```python
from build123d import *

# Parameters (mm, degrees)
F0_W     = 228.6
F0_H     = 88.9
F1_DEPTH = 1.27
F2_R     = 12.7
F4_DEPTH = 25.4
F6_DEPTH = 1.271


with BuildPart() as f1:
    # F0 (on Top) → F1 (new body)
    with BuildSketch(Plane.XY):
        with Locations((114.3, 44.45)):
            Rectangle(F0_W, F0_H)
    extrude(amount=F1_DEPTH)

    # F2
    f2_edges = [f1.edges().sort_by_distance(p)[0] for p in [
        (228.6, 0, 0.635),
        (228.6, 88.9, 0.635),
        (0, 88.9, 0.635),
        (0, 0, 0.635),
    ]]
    fillet(f2_edges, radius=F2_R)

    # F3 (on face) → F4 (cut)
    with BuildSketch(Plane.XY.offset(1.27)):
        with BuildLine():
            Line((44.45, 16.2687), (6.35, 16.2687))
            ThreePointArc((6.35, 16.2687), (2.7813, 12.7), (6.35, 9.1313))
            Line((6.35, 9.1313), (44.45, 9.1313))
            ThreePointArc((44.45, 9.1313), (48.0187, 12.7), (44.45, 16.2687))
        make_face()
        with BuildLine():
            ThreePointArc((6.35, 79.7687), (2.7813, 76.2), (6.35, 72.6313))
            Line((6.35, 72.6313), (44.45, 72.6313))
            ThreePointArc((44.45, 72.6313), (48.0187, 76.2), (44.45, 79.7687))
            Line((44.45, 79.7687), (6.35, 79.7687))
        make_face()
        with BuildLine():
            ThreePointArc((222.25, 72.6313), (225.8187, 76.2), (222.25, 79.7687))
            Line((222.25, 79.7687), (184.15, 79.7687))
            ThreePointArc((184.15, 79.7687), (180.5813, 76.2), (184.15, 72.6313))
            Line((184.15, 72.6313), (222.25, 72.6313))
        make_face()
        with BuildLine():
            ThreePointArc((222.25, 9.1313), (225.8187, 12.7), (222.25, 16.2687))
            Line((222.25, 16.2687), (184.15, 16.2687))
            ThreePointArc((184.15, 16.2687), (180.5813, 12.7), (184.15, 9.1313))
            Line((184.15, 9.1313), (222.25, 9.1313))
        make_face()
    extrude(amount=-F4_DEPTH, mode=Mode.SUBTRACT)

    # F5 (on face) → F6 (cut, through all)
    with BuildSketch(Plane.XY.offset(1.27)):
        with BuildLine():
            ThreePointArc((44.45, 63.5), (25.4, 44.45), (44.45, 25.4))
            Line((44.45, 25.4), (114.3, 25.4))
            Line((114.3, 25.4), (184.15, 25.4))
            ThreePointArc((184.15, 25.4), (203.2, 44.45), (184.15, 63.5))
            Line((184.15, 63.5), (114.3, 63.5))
            Line((114.3, 63.5), (44.45, 63.5))
        make_face()
    extrude(amount=-F6_DEPTH, mode=Mode.SUBTRACT)


solid = f1.part
```
Input: part model. Units: mm. Frame: model coordinates. A direction names the side the tool comes from. Round coordinates to 2 decimals unless told otherwise and drop trailing zeros. Loops run counter-clockwise (first coordinate to the right, second up) from the corner with the lowest first, then second, coordinate; pieces in that order, holes last. Notation, with made-up numbers: (62.25, 21) -> (104.25, 21) arc R20 ccw to (104.25, 37) -> close; hole circle Ø7 at (84.5, -20.75). An arc over 180 degrees is marked (long way). Use one line per item in the form item = value. Start each with the question number.
Item 1: Set-up query: faces 4 (the face through (203.195, 44.031, 0.644)), 5 (the face through (113, 25, 0)). Return all of +Z, -Z, +X, -X, +Y, -Y with unobstructed straight access to the full face (end or side cutting, diameter ignored); none if empty.
Item 2: Material intervals for L1, parallel to Y at x = 208.5, z = 1.2; L2, parallel to Y at x = 138, z = 0.15; L3, parallel to X at y = 74.5, z = 0.8, sorted ascending. Write a range as from..to.
Item 3: Section query C-C on z = 0.65. Return the cut outline in (x, y).
Item 4: Section query B-B on x = 205.5. Return the cut outline in (y, z), then the cut area to 3 significant figures.
Item 5: Section query D-D on y = 58. Return the cut outline in (x, z).
Item 6: Section query A-A on x = 59. Return the cut outline in (y, z), then the cut area to 3 significant figures.
Item 7: Contact query for a flat-ended pin moving along its axis: pin 1 Ø5 at (x, y) = (137, 23) entering from -Z. Output: stop coordinate, or through.
Item 8: Mould query, pull axis Y, two halves, no side actions, for faces 1 (the face through (3.62, 3.82, 0.64)), 2 (the face through (25.405, 44.869, 0.644)), 3 (the face through (3.62, 85.08, 0.64)). Classes: pulls with the +Y half, pulls with the -Y half, needs draft (parallel to the pull), parting line crosses it, or undercut.
Ans:
q1.face_4 = +Z, -Z
q1.face_5 = -Z, +X, -X, +Y, -Y
q2.L1 = 0..9.13, 16.27..72.63, 79.77..88.9
q2.L2 = 0..25.4, 63.5..88.9
q2.L3 = 0..3.21, 47.59..181.01, 225.39..228.6
q3.outline = (0, 12.7) arc R12.7 ccw to (12.7, 0) -> (215.9, 0) arc R12.7 ccw to (228.6, 12.7) -> (228.6, 76.2) arc R12.7 ccw to (215.9, 88.9) -> (12.7, 88.9) arc R12.7 ccw to (0, 76.2) -> close; hole (6.35, 9.13) -> (44.45, 9.13) arc R3.57 ccw to (44.45, 16.27) -> (6.35, 16.27) arc R3.57 ccw to start; hole (6.35, 72.63) -> (44.45, 72.63) arc R3.57 ccw to (44.45, 79.77) -> (6.35, 79.77) arc R3.57 ccw to start; hole (44.45, 25.4) -> (184.15, 25.4) arc R19.05 ccw to (184.15, 63.5) -> (44.45, 63.5) arc R19.05 ccw to start; hole (184.15, 9.13) -> (222.25, 9.13) arc R3.57 ccw to (222.25, 16.27) -> (184.15, 16.27) arc R3.57 ccw to start; hole (184.15, 72.63) -> (222.25, 72.63) arc R3.57 ccw to (222.25, 79.77) -> (184.15, 79.77) arc R3.57 ccw to start
q4.outline = (0, 0) -> (9.13, 0) -> (9.13, 1.27) -> (0, 1.27) -> close; (16.27, 0) -> (72.63, 0) -> (72.63, 1.27) -> (16.27, 1.27) -> close; (79.77, 0) -> (88.9, 0) -> (88.9, 1.27) -> (79.77, 1.27) -> close
q4.area = 94.8 mm^2
q5.outline = (0, 0) -> (31.06, 0) -> (31.06, 1.27) -> (0, 1.27) -> close; (197.54, 0) -> (228.6, 0) -> (228.6, 1.27) -> (197.54, 1.27) -> close
q6.outline = (0, 0) -> (25.4, 0) -> (25.4, 1.27) -> (0, 1.27) -> close; (63.5, 0) -> (88.9, 0) -> (88.9, 1.27) -> (63.5, 1.27) -> close
q6.area = 64.5 mm^2
q7.pin_1 = 0
q8.face_1 = pulls with the -Y half
q8.face_2 = undercut
q8.face_3 = pulls with the +Y half
